Answer from the drawing. Dimensions are ordinates in mm from the lowest x, y and z of the part. A direction names the side the tool comes from. Coordinates: 2 decimals unless noted, no trailing zeros. Loops run counter-clockwise (first coordinate to the right, second up) from the corner with the lowest first, then second, coordinate; pieces in that order, holes last. Notation, with made-up numbers: (62.25, 74.25) - (116.25, 74.25) arc R20 ccw to (116.25, 111.25) - close; hole circle Ø1 at (0.25, 52.5). An arc over 180 degrees is marked (long way). Write each question's results on one line, items separated by ' | '. Start each with the question number.
1. Each of these flat-tipped pins is pushed along its axis until it touches: P1, Ø1, axis at x = 5.5, z = 3.5, coming from the +Y side; P2, Ø1.6, axis at x = 3, y = 5, coming from the +Z side. Where does it stop, or does it pass through?
2. Find the intervals of material crossed by line 1 along X through (y, z) = (4.5, 1.75); line 2 along Z through (x, y) = (4, 2.5); line 3 along Y through (x, z) = (3.75, 3.85) (1 decimal), in increasing order. Write a range as [from, to].
3. Which of the six approach directions +Z, -Z, +X, -X, +Y, -Y give full straight-line access (tool end or side, diameter ignored) to the marked faces 1 and 2?
4. A cutting plane is placed at B-B on y = 20. Determine the outline of the cut face in (x, z), then the cut area to 3 significant figures.
5. A cutting plane is placed at D-D on z = 3. State how many separate pieces and enclosed holes the cut face has, then the cut area to 3 significant figures.
6. Determine the mould class of the marked faces 3, 4 and 5 for opening direction X: released by +X, released by -X, zero draft, split by the parting line, or undercut.
7. A cutting plane is placed at C-C on x = 5.25. Determine the outline of the cut face in (y, z) (1 decimal).
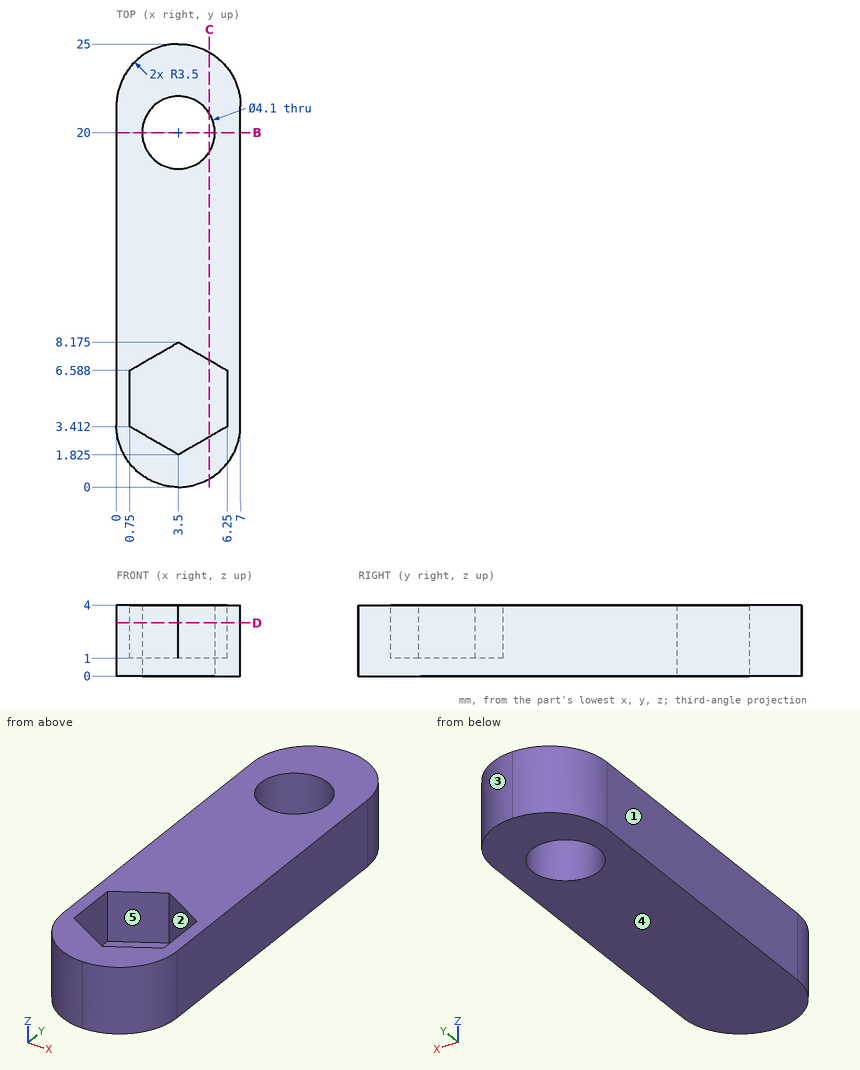
Values:
1) P1: y = 24.66 | P2: z = 1
2) line 1: [0, 0.75], [6.25, 7] | line 2: [0, 1] | line 3: [0, 2], [8, 18], [22, 25]
3) face 1: +Z, -Z, -X, +Y, -Y | face 2: +Z
4) outline: (0, 0) - (1.45, 0) - (1.45, 4) - (0, 4) - close; (5.55, 0) - (7, 0) - (7, 4) - (5.55, 4) - close | area: 11.6 mm^2
5) separate pieces: 1 | enclosed holes: 2 | area: 125 mm^2
6) face 3: released by +X | face 4: zero draft | face 5: undercut
7) outline: (0.5, 0) - (18.9, 0) - (18.9, 4) - (7.2, 4) - (7.2, 1) - (2.8, 1) - (2.8, 4) - (0.5, 4) - close; (21.1, 0) - (24.5, 0) - (24.5, 4) - (21.1, 4) - close
